CAD build for the part. Positions are in the model's coordinates, mm. A direction names the side the tool comes from. Round coordinates to 2 decimals unless told otherwise and drop trailing zeros. Write each loop counter-clockwise with the first axis right and the second up, starting at its lowest first coordinate (ties: lowest second). Pieces come first, ordered by that corner, then holes. Notation, with made-up numbers: (-30, 15.5) -> (8, 15.5) arc R34 cw to (8, 48.5) -> close; hole circle Ø7 at (63.25, -29.5). An arc over 180 degrees is marked (long way). Put each result on its own line as item: value. Start each with the question number.
1. Flat gauge pins, fed straight in: P1, Ø3, axis at x = 38.5, z = 1.5, coming from the -Y side; P2, Ø4, axis at x = 58, y = 30.5, coming from the +Z side; P3, Ø3.5, axis at x = 7.5, y = 7, coming from the +Z side. Where does each tip first touch, or does it go through?
2. Saw through at A-A on z = 4. State how many separate pieces and enclosed holes the cut face has, and give its area (3 significant figures).
3. Drill centre lines: line 1 (Y direction, x = 73.5, z = 2.7); line 2 (X direction, y = 18, z = 7.5); line 3 (Y direction, x = 55, z = 5.25). Where is each one in solid material? Low to high. Write a range as from..to.
4. Saw through at B-B on x = 22. List the corners of the cut face in (y, z).
5. Pull direction X, two halves, no side cores. Call faces 1 (the conical face through (1.733, 1.804, 0.171)), 2 (the flat face through (73, 54, 1)), 3 (the flat face through (80, 30, 4)): pulls with the +X half, pulls with the -X half, needs draft (parallel to the pull), parting line crosses it, or undercut.
6. 3-axis set-ups, long thin cutter, end or side, ignore diameter. For faces 4 (the conical face through (78.196, 1.733, 0.171)), 5 (the cylindrical face through (78, 2.06, 4.76)): which of +Z, -Z, +X, -X, +Y, -Y reach the whole face in a straight line?
7. Saw through at C-C on y = 34. List the corners of the cut face in (x, z), and give its area (3 significant figures).
Autodesk Inventor part; units mm, degrees
ref_plane "YZ Plane" through (0, 0, 0) normal (1, 0, 0) x (0, 1, 0)
ref_plane "XZ Plane" through (0, 0, 0) normal (0, 1, 0) x (-1, 0, 0)
ref_plane "XY Plane" through (0, 0, 0) normal (0, 0, 1) x (1, 0, 0)
sketch "Эскиз1" plane through (0, 0, 0) normal (0, 0, 1) x (1, 0, 0)
  line L0 (5, 0) -> (75, 0)
  line L1 (80, 5) -> (80, 55)
  line L2 (75, 60) -> (5, 60)
  line L3 (0, 55) -> (0, 5)
  arc A0 (5, 60) -> (0, 55) centre (5, 55) ccw
  arc A1 (80, 55) -> (75, 60) centre (75, 55) ccw
  arc A2 (0, 5) -> (5, 0) centre (5, 5) ccw
  arc A3 (75, 0) -> (80, 5) centre (75, 5) ccw
  point P0 (0, 0)
  point P1 (80, 60)
  point P2 (80, 0)
  point P3 (0, 60)
  dimension "d0" = 60
  dimension "d1" = 80
  dimension "d14" = 5
extrude "Выдавливание1" add sketch "Эскиз1" along normal blind 1
sketch "Эскиз2" plane through (0, 0, 1) normal (0, 0, 1) x (1, 0, 0)
  line L0 (80, 5) -> (80, 55)
  line L1 (75, 60) -> (5, 60)
  line L2 (0, 55) -> (0, 5)
  line L3 (5, 0) -> (75, 0)
  line L4 (0, 60) -> (0, 0)
  line L5 (0, 54) -> (80, 54) construction
  line L6 (80, 0) -> (80, 60)
  line L7 (0, 6) -> (80, 6) construction
  line L8 (6.5, 60) -> (6.5, 0) construction
  line L9 (0, 0) -> (80, 0)
  line L10 (80, 60) -> (0, 60)
  line L11 (73.5, 60) -> (73.5, 0) construction
  line L12 (0, 0) -> (80, 0)
  circle A0 centre (6.5, 54) radius 4
  circle A1 centre (73.5, 54) radius 4
  circle A2 centre (6.5, 6) radius 4
  circle A3 centre (73.5, 6) radius 4
  circle A4 centre (6.5, 54) radius 1.75
  circle A5 centre (73.5, 54) radius 1.75
  circle A6 centre (6.5, 6) radius 1.75
  circle A7 centre (73.5, 6) radius 1.75
  arc A8 (0, 5) -> (5, 0) centre (5, 5) ccw
  arc A9 (75, 0) -> (80, 5) centre (75, 5) ccw
  arc A10 (80, 55) -> (75, 60) centre (75, 55) ccw
  arc A11 (5, 60) -> (0, 55) centre (5, 55) ccw
  dimension "d4" = 48
  dimension "d5" = 67
  dimension "d6" = 6
  dimension "d7" = 6.5
  dimension "d8" = 8
  dimension "d10" = 3.5
extrude "Выдавливание2" add sketch "Эскиз2" along normal blind 6 contours A0 | A1 | A2 | A3
sketch "Эскиз3" plane through (0, 0, 1) normal (0, 0, 1) x (1, 0, 0)
  circle A0 centre (6.5, 6) radius 4
  circle A1 centre (73.5, 54) radius 4
  circle A2 centre (73.5, 6) radius 4
  circle A3 centre (6.5, 54) radius 4
  line L0 (0, 55) -> (0, 5)
  arc A4 (0, 5) -> (5, 0) centre (5, 5) ccw
  line L1 (5, 0) -> (75, 0)
  arc A5 (75, 0) -> (80, 5) centre (75, 5) ccw
  line L2 (80, 5) -> (80, 55)
  arc A6 (80, 55) -> (75, 60) centre (75, 55) ccw
  line L3 (75, 60) -> (5, 60)
  arc A7 (5, 60) -> (0, 55) centre (5, 55) ccw
  line L4 (5, 59.2) -> (75, 59.2)
  arc A8 (79.2, 55) -> (75, 59.2) centre (75, 55) ccw
  line L5 (79.2, 55) -> (79.2, 5)
  arc A9 (75, 0.8) -> (79.2, 5) centre (75, 5) ccw
  line L6 (75, 0.8) -> (5, 0.8)
  arc A10 (0.8, 5) -> (5, 0.8) centre (5, 5) ccw
  line L7 (0.8, 5) -> (0.8, 55)
  arc A11 (5, 59.2) -> (0.8, 55) centre (5, 55) ccw
  line L8 (6.5, 50) -> (0.8, 50)
  circle A12 centre (6.5, 54) radius 4
  line L9 (10.5, 54) -> (10.5, 59.2)
  line L10 (0.8, 10) -> (6.5, 10)
  circle A13 centre (6.5, 6) radius 4
  line L11 (10.5, 0.8) -> (10.5, 6)
  line L12 (69.5, 0.8) -> (69.5, 6)
  circle A14 centre (73.5, 6) radius 4
  circle A15 centre (73.5, 6) radius 4
  line L13 (73.5, 10) -> (79.2, 10)
  circle A16 centre (73.5, 54) radius 4
  line L14 (73.5, 50) -> (79.2, 50)
  line L15 (69.5, 59.2) -> (69.5, 54)
  point P0 (0, 0)
  dimension "d15" = 0.8
extrude "Выдавливание3" add sketch "Эскиз3" along normal blind 7
chamfer "Фаска1" distance 0.6 angle 45 24 edges at (40, 0, 0) (78.5355, 1.4645, 0) (80, 30, 0) (78.5355, 58.5355, 0) (40, 60, 0) (1.4645, 58.5355, 0) (0, 30, 0) (1.4645, 1.4645, 0) (40, 59.2, 1) (2.0302, 57.9698, 1) (0.8, 30, 1) (2.0302, 2.0302, 1) (40, 0.8, 1) (77.9698, 2.0302, 1) (79.2, 30, 1) (77.9698, 57.9698, 1) (4.75, 6, 7) (2.5, 6, 7) (4.75, 54, 7) (2.5, 54, 7) (71.75, 54, 7) (69.5, 54, 7) (71.75, 6, 7) (69.5, 6, 7)
properties part number "Корпус платы"
Return value:
1. P1: stops at y = 0
1. P2: stops at z = 1
1. P3: stops at z = 7
2. separate pieces: 5
2. enclosed holes: 5
2. area: 378 mm^2
3. line 1: y = 0..0.8, 2..4.25, 7.75..10, 50..52.25, 55.75..58, 59.2..60
3. line 2: x = 0..0.8, 79.2..80
3. line 3: y = 0..0.8, 59.2..60
4. outline: (0, 0.6) -> (0.6, 0) -> (59.4, 0) -> (60, 0.6) -> (60, 8) -> (59.2, 8) -> (59.2, 1.6) -> (58.6, 1) -> (1.4, 1) -> (0.8, 1.6) -> (0.8, 8) -> (0, 8) -> close
5. face 1: pulls with the -X half
5. face 2: undercut
5. face 3: pulls with the +X half
6. face 4: -Z, +X, -Y
6. face 5: +Z
7. outline: (0, 0.6) -> (0.6, 0) -> (79.4, 0) -> (80, 0.6) -> (80, 8) -> (79.2, 8) -> (79.2, 1.6) -> (78.6, 1) -> (1.4, 1) -> (0.8, 1.6) -> (0.8, 8) -> (0, 8) -> close
7. area: 91.2 mm^2
